from build123d import *

# Parameters (mm, degrees)
BOSS_EXTRUDE1_DEPTH = 5
SKETCH2_R           = 1.7
CUT_EXTRUDE1_DEPTH  = 36.05
CUT_EXTRUDE2_START  = 2
SKETCH3_R           = 3
CUT_EXTRUDE2_DEPTH  = 34.0500001
BOSS_EXTRUDE2_DEPTH = 5
SKETCH5_W           = 3.825
SKETCH5_H           = 24.9
CUT_EXTRUDE3_DEPTH  = 6
SKETCH6_W           = 5
SKETCH6_H           = 34.840664101
CUT_EXTRUDE4_DEPTH  = 32.2250001


with BuildPart() as part:
    # Sketch1 → Boss-Extrude1 (new body, symmetric)
    with BuildSketch(Plane.XY):
        with BuildLine():
            Line((-35.05, 0), (-10.15, 0))
            ThreePointArc((-10.15, 0), (0, 10.15), (10.15, 0))
            Line((10.15, 0), (35.05, 0))
            ThreePointArc((35.05, 0), (0, 35.05), (-35.05, 0))
        make_face()
    extrude(amount=BOSS_EXTRUDE1_DEPTH, both=True)

    # Sketch2 → Cut-Extrude1 (cut, through all)
    with BuildSketch(Plane(origin=(0, 0, 0), x_dir=(1, 0, 0), z_dir=(0, 1, 0))):
        with Locations((-25.05, 0)):
            Circle(SKETCH2_R)
    cut_extrude1 = extrude(amount=CUT_EXTRUDE1_DEPTH, mode=Mode.SUBTRACT)

    # Sketch3 → Cut-Extrude2 (cut, through all)
    with BuildSketch(Plane(origin=(0, 0, 0), x_dir=(1, 0, 0), z_dir=(0, 1, 0)).offset(CUT_EXTRUDE2_START)):
        with Locations((-25.05, 0)):
            Circle(SKETCH3_R)
    cut_extrude2 = extrude(amount=CUT_EXTRUDE2_DEPTH, mode=Mode.SUBTRACT)

    # Mirror1: Cut-Extrude1, Cut-Extrude2 across plane
    add(cut_extrude1.mirror(Plane(origin=(0, 0, 0), x_dir=(0, 0, 1), z_dir=(1, 0, 0))), mode=Mode.SUBTRACT)
    add(cut_extrude2.mirror(Plane(origin=(0, 0, 0), x_dir=(0, 0, 1), z_dir=(1, 0, 0))), mode=Mode.SUBTRACT)

    # Sketch4 → Boss-Extrude2 (add)
    with BuildSketch(Plane.XY.offset(5)):
        with BuildLine():
            Line((0, 12.5), (0, 35.05))
            ThreePointArc((0, 35.05), (24.784092681, 24.784092681), (35.05, 0))
            Line((35.05, 0), (12.5, 0))
            ThreePointArc((12.5, 0), (8.838834765, 8.838834765), (0, 12.5))
        make_face()
    boss_extrude2 = extrude(amount=BOSS_EXTRUDE2_DEPTH)

    # Sketch5 → Cut-Extrude3 (cut, through all)
    with BuildSketch(Plane.XY.offset(5)):
        with Locations((1.9125, 22.6)):
            Rectangle(SKETCH5_W, SKETCH5_H)
    cut_extrude3 = extrude(amount=CUT_EXTRUDE3_DEPTH, mode=Mode.SUBTRACT)

    # Mirror2: Boss-Extrude2, Cut-Extrude3 across plane
    add(boss_extrude2.mirror(Plane.XY))
    add(cut_extrude3.mirror(Plane.XY), mode=Mode.SUBTRACT)

    # Sketch6 → Cut-Extrude4 (cut, through all)
    with BuildSketch(Plane.ZY.offset(-3.825)):
        with Locations((7.5, 17.420332051)):
            Rectangle(SKETCH6_W, SKETCH6_H)
    extrude(amount=-CUT_EXTRUDE4_DEPTH, mode=Mode.SUBTRACT)


solid = part.part
Part model, mm, in its own coordinate system. A direction names the side the tool comes from. Give positions to 0.01 mm unless a question says otherwise; leave off trailing zeros. Loops run counter-clockwise (first coordinate to the right, second up) from the corner with the lowest first, then second, coordinate; pieces in that order, holes last.
(1) Band-saw the part on C-C (y = 23). Write the cut outline in (x, z) (3 decimals), and give its area (3 significant figures).
Return value:
outline: (-26.448, -5) - (3.825, -5) - (3.825, -10) - (26.448, -10) - (26.448, -2.654) arc R3 cw (long way) to (26.448, 2.654) - (26.448, 5) - (-26.448, 5) - (-26.448, 2.654) arc R3 cw (long way) to (-26.448, -2.654) - close
area: 598 mm2
(2) Pin check, flat tips, straight feed: pin 1 (17.5 mm diameter, centred on x = -0.5, y = 16.5, fed in from -Z); pin 2 (6 mm diameter, centred on x = 14.5, z = 0.5, fed in from +Y); pin 3 (5.5 mm diameter, centred on y = 26.5, z = -8, fed in from -X) (3 decimals); pin 4 (2 mm diameter, centred on x = 6.5, z = 3, fed in from -Y). Stop position of each tip, or through.
Return value:
pin 1: stops at z = -10
pin 2: stops at y = 33.11
pin 3: stops at x = 3.825
pin 4: stops at y = 6.84
(3) Band-saw the part on B-B (z = 0). Write the cut outline in (x, y), and give its area (3 significant figures).
Return value:
outline: (-35.05, 0) - (-26.75, 0) - (-26.75, 2) - (-28.05, 2) - (-28.05, 21.02) arc R35.05 ccw to start; (-23.35, 0) - (-10.15, 0) arc R10.15 cw to (10.15, 0) - (23.35, 0) - (23.35, 2) - (22.05, 2) - (22.05, 27.25) arc R35.05 ccw to (-22.05, 27.25) - (-22.05, 2) - (-23.35, 2) - close; (26.75, 0) - (35.05, 0) arc R35.05 ccw to (28.05, 21.02) - (28.05, 2) - (26.75, 2) - close
area: 1,490 mm2
(4) Band-saw the part on D-D (z = -9). Write the cut outline in (x, y) (3 decimals), and give its area (3 significant figures).
Return value:
outline: (3.825, 11.9) arc R12.5 cw to (12.5, 0) - (35.05, 0) arc R35.05 ccw to (3.825, 34.841) - close
area: 755 mm2
(5) Drill centre lines: line 1 along X through (y, z) = (0.4, 0); line 2 along Z through (x, y) = (-25, 18); line 3 along Z through (x, y) = (25.05, 1.05). Where is each one in solid material? Low to high.
Return value:
line 1: x = -35.05 to -26.75, -23.35 to -10.14, 10.14 to 23.35, 26.75 to 35.05
line 2: z = -5 to -3, 3 to 5
line 3: z = -10 to -1.7, 1.7 to 5
(6) Pull direction Z, two halves, no side cores. Call faces 4 (the cylindrical face through (22.28, 14.45, 1.15)), 5 (the flat face through (-17, 18, -5)), 6 (the cylindrical face through (-0.223, 10.148, 0.07)): pulls with the +Z half, pulls with the -Z half, needs draft (parallel to the pull), parting line crosses it, or undercut.
Return value:
face 4: undercut
face 5: pulls with the -Z half
face 6: needs draft
(7) Band-saw the part on A-A (x = -25.05). Write the cut outline in (y, z).
Return value:
outline: (0, -5) - (24.52, -5) - (24.52, -3) - (2, -3) - (2, -1.7) - (0, -1.7) - close; (0, 1.7) - (2, 1.7) - (2, 3) - (24.52, 3) - (24.52, 5) - (0, 5) - close
(8) 3-axis set-ups, long thin cutter, end or side, ignore diameter. For faces 1 (the flat face through (3.825, 23, -7)), 2 (the flat face through (23, 2, 0)), 3 (the cylindrical face through (10.17, 7.27, -7.46)): which of +Z, -Z, +X, -X, +Y, -Y reach the whole face in a straight line?
Return value:
face 1: -Z, -X, +Y, -Y
face 2: +Y
face 3: -Z, -X, -Y
